Verification items for the finished model (mm, model axes). A direction names the side the tool comes from. Give positions to 0.01 mm unless a question says otherwise; leave off trailing zeros. Write each loop counter-clockwise with the first axis right and the second up, starting at its lowest first coordinate (ties: lowest second). Pieces come first, ordered by that corner, then holes. Notation, with made-up numbers: M 65,22 L 123,22 A15 ccw 123,42 Z; hole C 45,6.5 d4. An arc over 180 degrees is marked long. Answer as a JSON object with one key per item and string values.
Autodesk Inventor part; units mm, degrees
ref_plane "작업 평면1" through (-15, -102.5, 52) normal (0, 0, -1) x (0, 1, 0)
ref_plane "작업 평면2" through (-7.15, 116.5, 9.5) normal (0, -1, 0) x (1, 0, 0)
ref_plane "YZ Plane" through (0, 0, 0) normal (1, 0, 0) x (0, 1, 0)
sketch "스케치1" plane through (0, 0, 0) normal (0, 0, 1) x (1, 0, 0)
  arc A0 (15, 100.5) -> (13, 102.5) centre (13, 100.5) ccw
  line L0 (13, 102.5) -> (-13, 102.5)
  arc A1 (-13, 102.5) -> (-15, 100.5) centre (-13, 100.5) ccw
  line L1 (-15, 100.5) -> (-15, -100.5)
  arc A2 (-15, -100.5) -> (-13, -102.5) centre (-13, -100.5) ccw
  line L2 (-13, -102.5) -> (-7, -102.5)
  arc A3 (-7, -102.5) -> (-5, -100.5) centre (-7, -100.5) ccw
  line L3 (-5, -100.5) -> (-5, -92.5)
  arc A4 (5, -92.5) -> (-5, -92.5) centre (0, -92.5) ccw
  line L4 (5, -92.5) -> (5, -100.5)
  arc A5 (5, -100.5) -> (7, -102.5) centre (7, -100.5) ccw
  line L5 (7, -102.5) -> (13, -102.5)
  arc A6 (13, -102.5) -> (15, -100.5) centre (13, -100.5) ccw
  line L6 (15, -100.5) -> (15, 100.5)
  circle A7 centre (7.7782, -100.2782) radius 1.25
  circle A8 centre (0, -81.5) radius 1.25
  circle A9 centre (-11, -92.5) radius 1.25
  circle A10 centre (11, -92.5) radius 1.25
  circle A11 centre (-7.7782, -100.2782) radius 1.25
  circle A12 centre (7.7782, -84.7218) radius 1.25
  circle A13 centre (-7.7782, -84.7218) radius 1.25
  circle A14 centre (-10.1627, 76.7095) radius 1.25
  circle A15 centre (-10.1627, 68.2905) radius 1.25
  circle A16 centre (10.1627, 68.2905) radius 1.25
  circle A17 centre (10.1627, 76.7095) radius 1.25
  circle A18 centre (4.2095, 82.6627) radius 1.25
  circle A19 centre (-4.2095, 82.6627) radius 1.25
  line L7 (0, 102.5) -> (0, 82.5)
  line L8 (15, 102.5) -> (-15, 102.5)
  line L9 (-15, 102.5) -> (-15, 62.5)
  line L10 (-15, 62.5) -> (15, 62.5)
  line L11 (15, 62.5) -> (15, 102.5)
  line L12 (15, 102.5) -> (-15, 62.5) construction
  line L13 (-15, 102.5) -> (15, 62.5) construction
  point P0 (0, 0)
  dimension "d0" = 20
  dimension "d1" = 40
ref_plane "작업 평면1" through (-15, -102.5, 52) normal (0, 0, -1) x (0, 1, 0)
extrude "돌출1" add sketch "스케치1" along normal up to surface (52 mm away) contours L6 L10 L1 A1 L0 A0
sketch "스케치2" plane through (-13, 102.5, 0) normal (0, 1, 0) x (1, 0, 0)
  line L0 (-0.4121, -11.5) -> (26.4121, -11.5)
  line L1 (-0.4121, -45.5) -> (26.4121, -45.5)
  line L2 (-2, 0) -> (-2, -52)
  line L3 (28, 0) -> (28, -52)
  line L4 (-2, -52) -> (28, -52)
  line L5 (28, -52) -> (28, -45.5)
  line L6 (28, -45.5) -> (-2, -45.5)
  line L7 (-2, -45.5) -> (-2, -52)
  line L8 (-2, 0) -> (28, 0)
  line L9 (28, 0) -> (28, -11.5)
  line L10 (28, -11.5) -> (-2, -11.5)
  line L11 (-2, -11.5) -> (-2, 0)
  point P0 (13, 0)
  dimension "d4" = 30
ref_plane "작업 평면2" through (-7.15, 116.5, 9.5) normal (0, -1, 0) x (1, 0, 0)
extrude "돌출2" add sketch "스케치2" along normal up to surface (14 mm away) contours L10 L2 L8 L3 L0 | L6 L1 L3 L4 L2
sketch "스케치3" plane through (0, 0, 0) normal (0, 0, -1) x (-1, 0, 0)
  line L0 (-15, 102.5) -> (-13, 102.5)
  line L1 (-15, 62.5) -> (-15, 100.5)
  line L2 (-15, 102.5) -> (-15, 100.5)
  line L3 (15, 100.5) -> (15, 62.5)
  line L4 (-15, 100.5) -> (15, 100.5)
  line L5 (15, 100.5) -> (15, 102.5)
  arc A0 (15, 100.5) -> (13, 102.5) centre (13, 100.5) ccw
  line L6 (-15, 102.5) -> (15, 102.5)
  line L7 (13, 102.5) -> (-13, 102.5)
  point P0 (0, 0)
extrude "돌출3" add sketch "스케치3" against normal up to surface (52 mm away)
sketch "스케치4" plane through (0, 0, 0) normal (0, 0, -1) x (-1, 0, 0)
  circle A0 centre (-17.3, 119) radius 1.35
  circle A1 centre (17.3, 119) radius 1.35
  line L0 (-20.1, 119.3234) -> (-20.1, 163.5766)
  arc A2 (-20.1, 119.3234) -> (-19.5808, 117.6364) centre (-17.1, 119.3234) ccw
  line L1 (-15.8929, 112.2131) -> (-19.5808, 117.6364)
  arc A3 (-15.8929, 112.2131) -> (-13.4121, 110.9) centre (-13.4121, 113.9) ccw
  line L2 (13.4121, 110.9) -> (-13.4121, 110.9)
  arc A4 (13.4121, 110.9) -> (15.8929, 112.2131) centre (13.4121, 113.9) ccw
  line L3 (19.5808, 117.6364) -> (15.8929, 112.2131)
  arc A5 (19.5808, 117.6364) -> (20.1, 119.3234) centre (17.1, 119.3234) ccw
  line L4 (20.1, 163.5766) -> (20.1, 119.3234)
  arc A6 (20.1, 163.5766) -> (19.5808, 165.2636) centre (17.1, 163.5766) ccw
  line L5 (15.5953, 171.1246) -> (19.5808, 165.2636)
  arc A7 (15.5953, 171.1246) -> (13.9414, 172) centre (13.9414, 170) ccw
  line L6 (6.65, 172) -> (13.9414, 172)
  arc A8 (8.15, 170.5) -> (6.65, 172) centre (6.65, 170.5) ccw
  line L7 (8.15, 170.5) -> (8.15, 168)
  arc A9 (8.15, 168) -> (10.5, 165.65) centre (10.5, 168) ccw
  line L8 (10.5, 165.65) -> (13.5, 165.65)
  arc A10 (14.5, 164.65) -> (13.5, 165.65) centre (13.5, 164.65) ccw
  line L9 (14.5, 164.65) -> (14.5, 123.85)
  arc A11 (13.5, 122.85) -> (14.5, 123.85) centre (13.5, 123.85) ccw
  line L10 (13.5, 122.85) -> (10.5, 122.85)
  arc A12 (10.5, 122.85) -> (8.15, 120.5) centre (10.5, 120.5) ccw
  line L11 (8.15, 120.5) -> (8.15, 117.5)
  arc A13 (7.15, 116.5) -> (8.15, 117.5) centre (7.15, 117.5) ccw
  line L12 (7.15, 116.5) -> (-7.15, 116.5)
  arc A14 (-8.15, 117.5) -> (-7.15, 116.5) centre (-7.15, 117.5) ccw
  line L13 (-8.15, 117.5) -> (-8.15, 120.5)
  arc A15 (-8.15, 120.5) -> (-10.5, 122.85) centre (-10.5, 120.5) ccw
  line L14 (-10.5, 122.85) -> (-13.5, 122.85)
  arc A16 (-14.5, 123.85) -> (-13.5, 122.85) centre (-13.5, 123.85) ccw
  line L15 (-14.5, 123.85) -> (-14.5, 164.65)
  arc A17 (-13.5, 165.65) -> (-14.5, 164.65) centre (-13.5, 164.65) ccw
  line L16 (-13.5, 165.65) -> (-10.5, 165.65)
  arc A18 (-10.5, 165.65) -> (-8.15, 168) centre (-10.5, 168) ccw
  line L17 (-8.15, 168) -> (-8.15, 170.5)
  arc A19 (-6.65, 172) -> (-8.15, 170.5) centre (-6.65, 170.5) ccw
  line L18 (-13.9414, 172) -> (-6.65, 172)
  arc A20 (-13.9414, 172) -> (-15.5953, 171.1246) centre (-13.9414, 170) ccw
  line L19 (-19.5808, 165.2636) -> (-15.5953, 171.1246)
  arc A21 (-19.5808, 165.2636) -> (-20.1, 163.5766) centre (-17.1, 163.5766) ccw
  arc A22 (15.95, 163) -> (18.65, 163) centre (17.3, 163) ccw
  arc A23 (18.65, 163) -> (15.95, 163) centre (17.3, 163) ccw
  arc A24 (15.95, 141) -> (18.65, 141) centre (17.3, 141) ccw
  arc A25 (18.65, 141) -> (15.95, 141) centre (17.3, 141) ccw
  arc A26 (9.65, 113.7) -> (12.35, 113.7) centre (11, 113.7) ccw
  arc A27 (12.35, 113.7) -> (9.65, 113.7) centre (11, 113.7) ccw
  arc A28 (-18.65, 163) -> (-15.95, 163) centre (-17.3, 163) ccw
  arc A29 (-15.95, 163) -> (-18.65, 163) centre (-17.3, 163) ccw
  arc A30 (-18.65, 141) -> (-15.95, 141) centre (-17.3, 141) ccw
  arc A31 (-15.95, 141) -> (-18.65, 141) centre (-17.3, 141) ccw
  arc A32 (-12.35, 113.7) -> (-9.65, 113.7) centre (-11, 113.7) ccw
  arc A33 (-9.65, 113.7) -> (-12.35, 113.7) centre (-11, 113.7) ccw
  point P0 (0, 0)
extrude "돌출4" cut sketch "스케치4" against normal through all contours A27 A26 | A33 A32
properties part number "link"
1) Thickness scan on L1, parallel to Y at x = 10, z = 32; L2, parallel to X at y = 113.7, z = 49; L3, parallel to Y at x = 9.5, z = 50. Record the ranges inside material, lowest first.
Completed:
{"L1": "y = 62.5 to 67.05, 69.53 to 75.47, 77.95 to 102.5", "L2": "x = -15 to -12.35, -9.65 to 9.65, 12.35 to 15", "L3": "y = 62.5 to 67.23, 69.35 to 75.65, 77.77 to 116.5"}
2) Section check A-A on y = 113.7. Record the boundary of the cut face in (x, z), and give its area (3 significant figures).
Completed:
{"outline": "M -15,0 L -12.35,0 L -12.35,11.5 L -15,11.5 Z; M -15,45.5 L -12.35,45.5 L -12.35,52 L -15,52 Z; M -9.65,0 L 9.65,0 L 9.65,11.5 L -9.65,11.5 Z; M -9.65,45.5 L 9.65,45.5 L 9.65,52 L -9.65,52 Z; M 12.35,0 L 15,0 L 15,11.5 L 12.35,11.5 Z; M 12.35,45.5 L 15,45.5 L 15,52 L 12.35,52 Z", "area": "443 mm2"}
3) Section check C-C on x = -10.5. Record the boundary of the cut face in (y, z).
Completed:
{"outline": "M 62.5,0 L 67.09,0 L 67.09,52 L 62.5,52 Z; M 69.49,0 L 75.51,0 L 75.51,52 L 69.49,52 Z; M 77.91,0 L 112.45,0 L 112.45,11.5 L 102.5,11.5 L 102.5,45.5 L 112.45,45.5 L 112.45,52 L 77.91,52 Z; M 114.95,0 L 116.5,0 L 116.5,11.5 L 114.95,11.5 Z; M 114.95,45.5 L 116.5,45.5 L 116.5,52 L 114.95,52 Z"}
4) Access from +Z, -Z, +X, -X, +Y, -Y to the whole of each face (thin tool, end or side, straight path). Record for faces 1 (the face through (0, 109, 11.5)), 2 (the face through (-3.63, 83.77, 25.64)).
Completed:
{"face 1": "+X, -X, +Y", "face 2": "+Z, -Z"}
5) Section check D-D on z = 47. Count the separate pieces of the cut face and the enclosed holes in it, and give its area (3 significant figures).
Completed:
{"separate pieces": "1", "enclosed holes": "8", "area": "1,580 mm2"}
6) Go/stop test with a flat-tipped pin: pin 1 (1 mm diameter, centred on x = -2.5, z = 44, fed in from +Y). Record where the tip stops, or that it passes through.
Completed:
{"pin 1": "stops at y = 102.5"}
7) Release check for a two-part mould opening along X. For faces 3 (the face through (0, 109, 45.5)), 4 (the face through (15, 83, 26)), 5 (the face through (-9.59, 77.82, 25.64)) record: pulls with the +X half, pulls with the -X half, needs draft (parallel to the pull), parting line crosses it, or undercut.
Completed:
{"face 3": "needs draft", "face 4": "pulls with the +X half", "face 5": "undercut"}
8) Section check B-B on y = 107. Record the boundary of the cut face in (x, z).
Completed:
{"outline": "M -15,0 L 15,0 L 15,11.5 L -15,11.5 Z; M -15,45.5 L 15,45.5 L 15,52 L -15,52 Z"}
